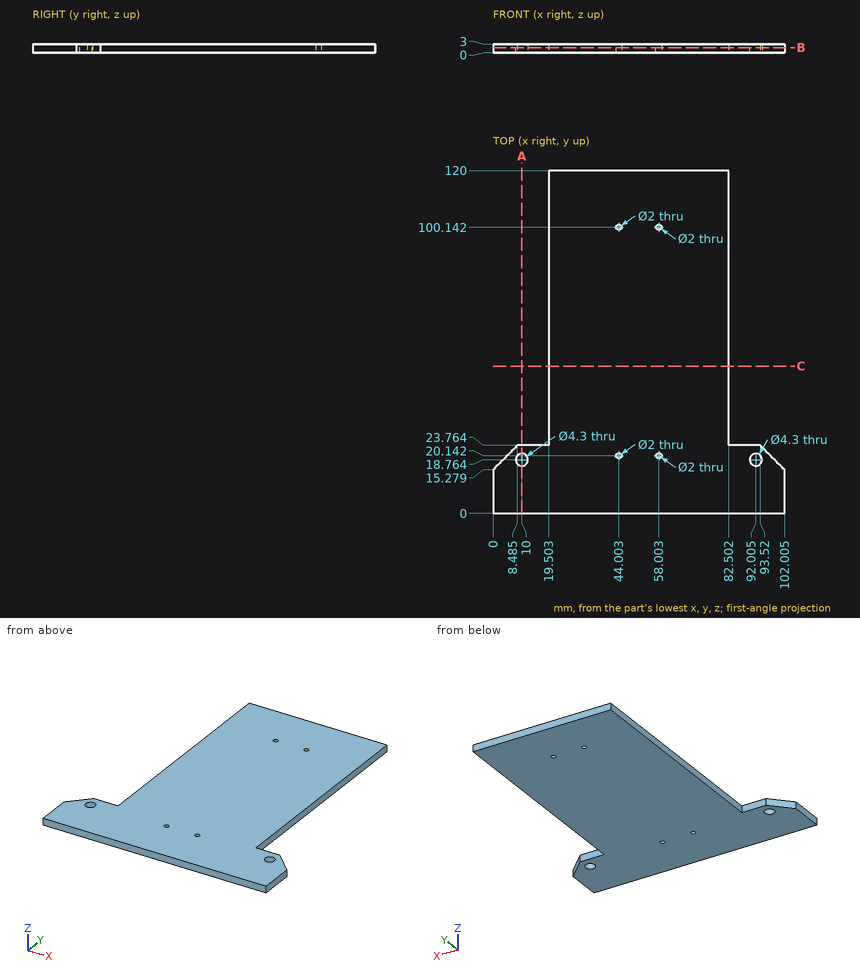
Drawing for the job (mm, zero at the part's lowest x, y, z). Coordinates: 2 decimals unless noted, no trailing zeros. Write each loop counter-clockwise with the first axis right and the second up, starting at its lowest first coordinate (ties: lowest second). Pieces come first, ordered by that corner, then holes. Notation, with made-up numbers: (83, -16.75) -> (110, -16.75) arc R26 cw to (110, 3.25) -> close; hole circle Ø5 at (78, 84.5). An arc over 180 degrees is marked (long way). One line per item, written item: value. Start each with the question number.
1) Slice it at C-C on y = 51.5. Write the cut outline in (x, z).
2) Flat gauge pins, fed straight in: pin 1 Ø7 at (x, y) = (10, 18.76) entering from +Z; pin 2 Ø1.2 at (x, y) = (44, 100.14) entering from +Z; pin 3 Ø1 at (y, z) = (107.5, 0.5) entering from -X. Where does each tip first touch, or does it go through?
3) Slice it at A-A on x = 10. Write the cut outline in (y, z) (1 decimal).
4) Slice it at B-B on z = 1.7. Count the separate pieces of the cut face and the enclosed holes in it, then the cut area to 3 significant figures.
5) Probe probe 1 along X at (y, z) = (43, 2.6); probe 2 along Y at (x, z) = (10.5, 0.9) (1 decimal); probe 3 along Y at (x, z) = (10, 1.7) (1 decimal). List the from-to ranges inside material, lowest first.
Answers follow:
1. outline: (19.5, 0) -> (82.5, 0) -> (82.5, 3) -> (19.5, 3) -> close
2. pin 1: z = 3
2. pin 2: through
2. pin 3: x = 19.5
3. outline: (0, 0) -> (16.6, 0) -> (16.6, 3) -> (0, 3) -> close; (20.9, 0) -> (23.8, 0) -> (23.8, 3) -> (20.9, 3) -> close
4. separate pieces: 1
4. enclosed holes: 6
4. area: 8,370 mm2
5. probe 1: 19.5 to 82.5
5. probe 2: 0 to 16.7, 20.9 to 23.8
5. probe 3: 0 to 16.6, 20.9 to 23.8
